Design review of the part built by this model. Coordinates are the model's own, in mm. Face numbers are marked on the shaded views. A direction names the side the tool comes from. Give positions to 0.01 mm unless a question says otherwise; leave off trailing zeros. Write each loop counter-clockwise with the first axis right and the second up, starting at its lowest first coordinate (ties: lowest second). Pieces come first, ordered by that corner, then holes. Notation, with made-up numbers: M 10.25,-4 L 51.25,-4 A22 ccw 51.25,18 Z; hole C 45.25,-8.75 d7. An arc over 180 degrees is marked long. Write each question's results on one line, items separated by ' | '. Start each with the question number.
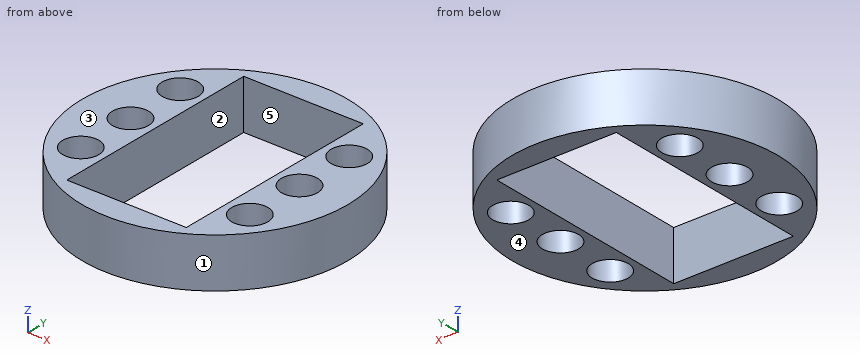
Autodesk Inventor part; units mm, degrees
ref_plane "YZ Plane" through (0, 0, 0) normal (1, 0, 0) x (0, 1, 0)
ref_plane "XZ Plane" through (0, 0, 0) normal (0, 1, 0) x (-1, 0, 0)
ref_plane "XY Plane" through (0, 0, 0) normal (0, 0, 1) x (1, 0, 0)
sketch "Sketch3" plane through (0, 0, 0) normal (0, 0, 1) x (1, 0, 0)
  line L0 (-15.8918, -16.7) -> (15.8918, -16.7)
  line L1 (16.7, -15.7) -> (16.7, 15.7)
  line L2 (15.8918, 16.7) -> (-15.8918, 16.7)
  line L3 (-16.7, 15.7) -> (-16.7, -15.7)
  line L4 (-15.8918, 16.7) -> (-16.7, 15.7)
  line L5 (15.8918, 16.7) -> (16.7, 15.7)
  line L6 (16.7, -15.7) -> (15.8918, -16.7)
  line L7 (-16.7, -15.7) -> (-15.8918, -16.7)
  line L8 (-4.9497, -8.8994) -> (4.9497, -8.8994)
  line L9 (4.9497, -8.8994) -> (4.9497, 8.8994)
  line L10 (4.9497, 8.8994) -> (-4.9497, 8.8994)
  line L11 (-4.9497, 8.8994) -> (-4.9497, -8.8994)
  circle A0 centre (-12.14, 12.625) radius 2.045
  circle A1 centre (12.14, 12.625) radius 2.045
  line L12 (0, -16.7) -> (0, 16.7) construction
  circle A2 centre (-12.14, -12.625) radius 2.045
  circle A3 centre (12.14, -12.625) radius 2.045
  line L13 (12.14, 12.625) -> (-12.14, 12.625) construction
  line L14 (-12.14, 12.625) -> (-12.14, -12.625) construction
  line L15 (-12.14, -12.625) -> (12.14, -12.625) construction
  line L16 (12.14, -12.625) -> (12.14, 12.625) construction
  line L17 (-16.7, 0) -> (16.7, 0) construction
  circle A4 centre (0, 0) radius 18.4 construction
  circle A5 centre (-7, 0) radius 1.5
  circle A6 centre (7, 0) radius 1.5
  circle A7 centre (-7, 5) radius 1.5
  circle A8 centre (7, 5) radius 1.5
  circle A9 centre (-7, -5) radius 1.5
  circle A10 centre (7, -5) radius 1.5
  dimension "d10" = 9.8994
  dimension "d11" = 17.7988
  dimension "d12" = 4.09
  dimension "d13" = 4.09
  dimension "d17" = 4.09
  dimension "d19" = 24.28
  dimension "d20" = 25.25
  dimension "d21" = 4.09
  dimension "d22" = 12.625
  dimension "d26" = 36.8
  dimension "d38" = 12.14
  dimension "d39" = 33.4
  dimension "d40" = 33.4
  dimension "d41" = 3
  dimension "d42" = 3
  dimension "d43" = 7
  dimension "d44" = 7
  dimension "d45" = 3
  dimension "d46" = 3
  dimension "d47" = 3
  dimension "d48" = 3
  dimension "d49" = 5
  dimension "d50" = 5
  dimension "d51" = 5
  dimension "d52" = 5
  dimension "d57" = 8.8994
  dimension "d58" = 4.9497
sketch "Sketch4" plane through (0, 0, 0) normal (0, 0, 1) x (1, 0, 0)
  circle A0 centre (0, 0) radius 11
  dimension "d32" = 22
extrude "Extrusion5" add sketch "Sketch3" along normal blind 4.1
extrude "Extrusion6" cut sketch "Sketch4" along normal blind 4.1 keep common part
properties part number "WG18FLANGECutDown" material "Brass, Soft Yellow"
Q1. For pin 1 Ø2 at (y, z) = (2, 3) entering from +X; pin 2 Ø1.5 at (x, z) = (3, 0.5) entering from +Y; pin 3 Ø1.2 at (x, z) = (-1.5, 2) entering from -Y; pin 4 Ø2.5 at (x, y) = (-7, 5) entering from -Z, all flat-tipped, find the tip position at first contact; note any pin that passes through.
Q2. We need section B-B on x = 7.5. Write out the cut boundary in (y, z).
Q3. For the marked faces 4 and 5, list the 3-axis set-ups (+Z, -Z, +X, -X, +Y, -Y) from which the entire face can be reached by the end or side of a thin tool; tool diameter is ignored.
Q4. Wall thickness on line 1 along X through (y, z) = (-6, 3.8); line 2 along X through (y, z) = (-1, 0.6); line 3 along Y through (x, z) = (-7, 1.6): over which ranges is each line inside the solid? List them lowest first. Write a range as from..to.
Q5. We need section A-A on z = 1.4. Write out the cut boundary in (x, y).
Q6. We need section C-C on y = -2.75. Write out the cut boundary in (x, z), and give its area (3 significant figures).
Q7. The part is to be moulded in two halves that separate along X. For the marked faces 1, 2 and 3, say which applies: pulls with the +X half, pulls with the -X half, needs draft (parallel to the pull), parting line crosses it, or undercut.
Q8. We need section D-D on x = 2.25. Write out the cut boundary in (y, z), and give its area (3 significant figures).
Answer sheet:
1) pin 1: x = 10.95 | pin 2: y = 10.77 | pin 3: y = -10.96 | pin 4: through
2) outline: M -8.05,0 L -6.41,0 L -6.41,4.1 L -8.05,4.1 Z; M -3.59,0 L -1.41,0 L -1.41,4.1 L -3.59,4.1 Z; M 1.41,0 L 3.59,0 L 3.59,4.1 L 1.41,4.1 Z; M 6.41,0 L 8.05,0 L 8.05,4.1 L 6.41,4.1 Z
3) face 4: -Z, +X, -X, +Y, -Y | face 5: +Z, -Z
4) line 1: -9.22..-8.12, -5.88..-4.95, 4.95..5.88, 8.12..9.22 | line 2: -10.95..-8.12, -5.88..-4.95, 4.95..5.88, 8.12..10.95 | line 3: -8.49..-6.5, -3.5..-1.5, 1.5..3.5, 6.5..8.49
5) outline: C 0,0 d22; hole C -7,-5 d3; hole C -7,0 d3; hole C -7,5 d3; hole M -4.95,-8.9 L 4.95,-8.9 L 4.95,8.9 L -4.95,8.9 Z; hole C 7,-5 d3; hole C 7,0 d3; hole C 7,5 d3
6) outline: M -10.65,0 L -4.95,0 L -4.95,4.1 L -10.65,4.1 Z; M 4.95,0 L 10.65,0 L 10.65,4.1 L 4.95,4.1 Z | area: 46.7 mm^2
7) face 1: parting line crosses it | face 2: undercut | face 3: needs draft
8) outline: M -10.77,0 L -8.9,0 L -8.9,4.1 L -10.77,4.1 Z; M 8.9,0 L 10.77,0 L 10.77,4.1 L 8.9,4.1 Z | area: 15.3 mm^2
